Geometry: see drawing. Coordinates: mm, zero at the bounding-box minimum. A direction names the side the tool comes from. Round coordinates to 2 decimals unless told otherwise and drop trailing zeros. Loops run counter-clockwise (first coordinate to the right, second up) from the corner with the lowest first, then second, coordinate; pieces in that order, holes last.
(1) Cut plane C-C, the plane y = 3.4. Output: boundary loops of the cut face in (x, z).
(2) Line query: line 1 (X direction, y = 3.3, z = 3); line 2 (Z direction, x = 2.25, y = 1.9). Output: solid intervals per line, ascending.
(3) Cut plane A-A, the plane z = 3. Output: boundary loops of the cut face in (x, y), and give its area (3 significant figures).
(4) Access query for the marked faces 1 and 2. Directions: +Z, -Z, +X, -X, +Y, -Y. A direction counts if a zero-diameter tool reaches every point of the face in a straight line with its end or side. Return the directions, or none.
(5) Draft query along Z for the marked faces 3, 4 and 5. Return one class per face: released by +Z, released by -Z, zero draft, split by the parting line, or undercut.
(6) First-contact query: pin 1 Ø1.5 at (x, y) = (2.5, 1) entering from -Z; pin 2 Ø1.5 at (x, y) = (5, 1) entering from +Z; pin 3 Ø1 at (x, y) = (1, 1.5) entering from -Z. Flat tips, straight axial feed; report the tip coordinate or a pass-through.
(7) Cut plane B-B, the plane x = 3. Output: boundary loops of the cut face in (y, z), and give its area (3 significant figures).
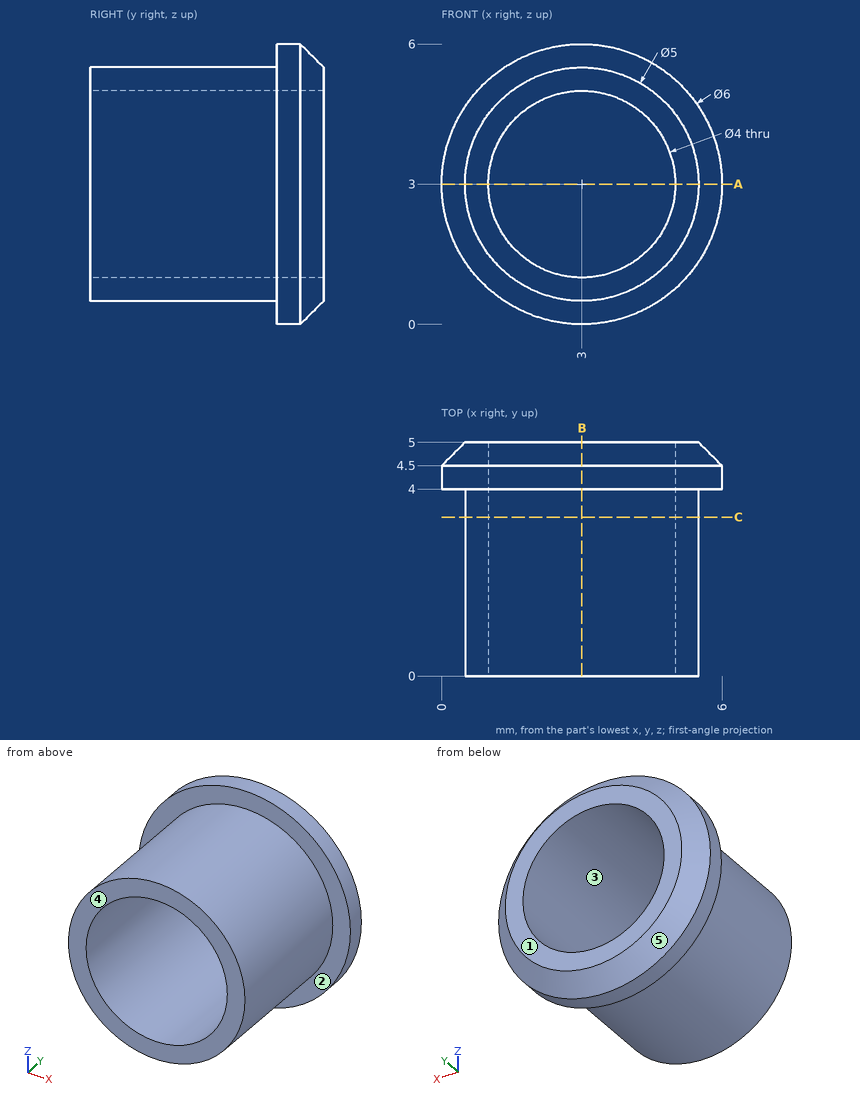
Reported:
1. outline: circle Ø5 at (3, 3); hole circle Ø4 at (3, 3)
2. line 1: x = 0.5 to 1, 5 to 5.5
2. line 2: z = 0.62 to 1.15, 4.85 to 5.38
3. outline: (0, 4) - (0.5, 4) - (0.5, 0) - (1, 0) - (1, 5) - (0.5, 5) - (0, 4.5) - close; (5, 0) - (5.5, 0) - (5.5, 4) - (6, 4) - (6, 4.5) - (5.5, 5) - (5, 5) - close
3. area: 5.75 mm2
4. face 1: +Z, -Z, +X, -X, +Y
4. face 2: -Y
5. face 3: undercut
5. face 4: zero draft
5. face 5: split by the parting line
6. pin 1: stops at z = 0.5
6. pin 2: stops at z = 5.17
6. pin 3: stops at z = 1
7. outline: (0, 0.5) - (4, 0.5) - (4, 0) - (4.5, 0) - (5, 0.5) - (5, 1) - (0, 1) - close; (0, 5) - (5, 5) - (5, 5.5) - (4.5, 6) - (4, 6) - (4, 5.5) - (0, 5.5) - close
7. area: 5.75 mm2
